CAD build for the part. Positions are in the model's coordinates, mm. Face numbers are marked on the shaded views. A direction names the side the tool comes from. Give positions to 0.01 mm unless a question says otherwise; leave off trailing zeros. Order: outer loops, then holes, each group sorted by start corner. A loop starts at its lowest first (then second) coordinate and runs counter-clockwise, first axis right, second up.
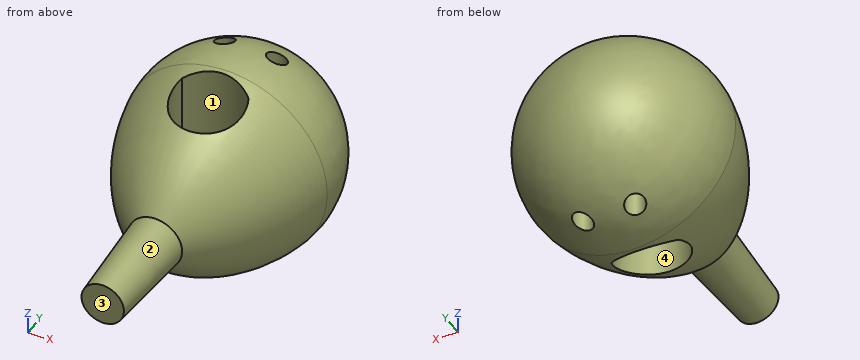
```python
from build123d import *

# Parameters (mm, degrees)
F2_R     = 4
F3_DEPTH = 41.765352
F4_DEPTH = 41.765352


with BuildPart() as f1:
    # F0 (on Top) → F1 (revolve)
    with BuildSketch(Plane.XY):
        Polygon((0, -39.931846), (0, 0), (-11, 0), (-8.665983, -39.931846), align=None)
        with BuildLine():
            Line((-11, 0), (0, 0))
            Line((0, 0), (0, 100.485936))
            ThreePointArc((0, 100.485936), (-31.287978, 86.386065), (-41.449975, 53.606838))
            ThreePointArc((-41.449975, 53.606838), (-31.054628, 24.060067), (-11, 0))
        make_face()
    revolve(axis=Axis((0, 50.242968, 0), (0, -1, 0)))

    # F2 (on Top) → F3 (cut, through all)
    with BuildSketch(Plane.XY):
        with Locations((10.89077, 72.268995)):
            Circle(F2_R)
        with Locations((-10.376575, 72.137559)):
            Circle(F2_R)
        with BuildLine():
            ThreePointArc((12.932606, 46.952406), (-0.683245, 51.822724), (-14.113051, 46.460665))
            ThreePointArc((-14.113051, 46.460665), (-0.224508, 26.592261), (12.932606, 46.952406))
        make_face()
    extrude(amount=-F3_DEPTH, mode=Mode.SUBTRACT)

    # F2 (on Top) → F4 (cut, through all)
    with BuildSketch(Plane.XY):
        with Locations((10.89077, 72.268995)):
            Circle(F2_R)
        with Locations((-10.376575, 72.137559)):
            Circle(F2_R)
        with BuildLine():
            ThreePointArc((12.932606, 46.952406), (-0.683245, 51.822724), (-14.113051, 46.460665))
            ThreePointArc((-14.113051, 46.460665), (-0.224508, 26.592261), (12.932606, 46.952406))
        make_face()
    extrude(amount=F4_DEPTH, mode=Mode.SUBTRACT)


solid = f1.part
```
Item 1: Drop flat-ended pins along their axis: pin 1 Ø9 at (x, y) = (-10.38, 72.14) entering from -Z; pin 2 Ø8 at (x, z) = (32, 16.5) entering from +Y; pin 3 Ø12 at (x, z) = (-18.5, -26) entering from +Y. Give the stop position or say it passes through.
Item 2: Tool access for the marked faces 1 and 2: list every direction of +Z, -Z, +X, -X, +Y, -Y with a clear straight run to the whole face (end or side of a thin tool).
Item 3: Slice it at C-C (y = -17). Give the cut face in (x, z), and give its area (3 significant figures).
Item 4: Two-plate mould, pull along Y, no slides. Class the marked faces 3 and 4: released by +Y, released by -Y, zero draft, split by the parting line, or undercut.
Item 5: Slice it at A-A (z = -3). State how many separate pieces and enclosed holes the cut face has, and give its area (3 significant figures).
Item 6: Wall check: L1, parallel to X at y = 73, z = -19; L2, parallel to X at y = 75, z = -6.5; L3, parallel to Y at x = 12, z = -11. Give the ranges that are in metal, low to high.
A:
1. pin 1: stops at z = -39.86
1. pin 2: stops at y = 85.56
1. pin 3: stops at y = 91.48
2. face 1: +Z, -Z
2. face 2: -Y
3. outline: circle Ø20.01 at (0, 0)
3. area: 315 mm2
4. face 3: released by -Y
4. face 4: undercut
5. separate pieces: 1
5. enclosed holes: 3
5. area: 6,460 mm2
6. L1: x = -34.34 to -14.28, -6.47 to 6.96, 14.82 to 34.34
6. L2: x = -37.91 to -13.17, -7.58 to 7.97, 13.81 to 37.91
6. L3: y = 4.8 to 33.62, 47.7 to 68.43, 76.11 to 97.18
